Geometry check sheet. Reference: drawing and pictorial views, mm from the part's lowest x, y, z. Round coordinates to 2 decimals unless told otherwise and drop trailing zeros. Write each loop counter-clockwise with the first axis right and the second up, starting at its lowest first coordinate (ties: lowest second). Pieces come first, ordered by that corner, then holes.
Item 1: Section check B-B, the plane x = 14. Record the cut outline in (y, z) (1 decimal), plus the area to 3 significant figures.
Item 2: Section check C-C, the plane y = 65.5. State how many separate pieces and enclosed holes the cut face has.
Item 3: Material ranges on line 1 along Y through (x, z) = (19, 2.6) (1 decimal), recorded low to high.
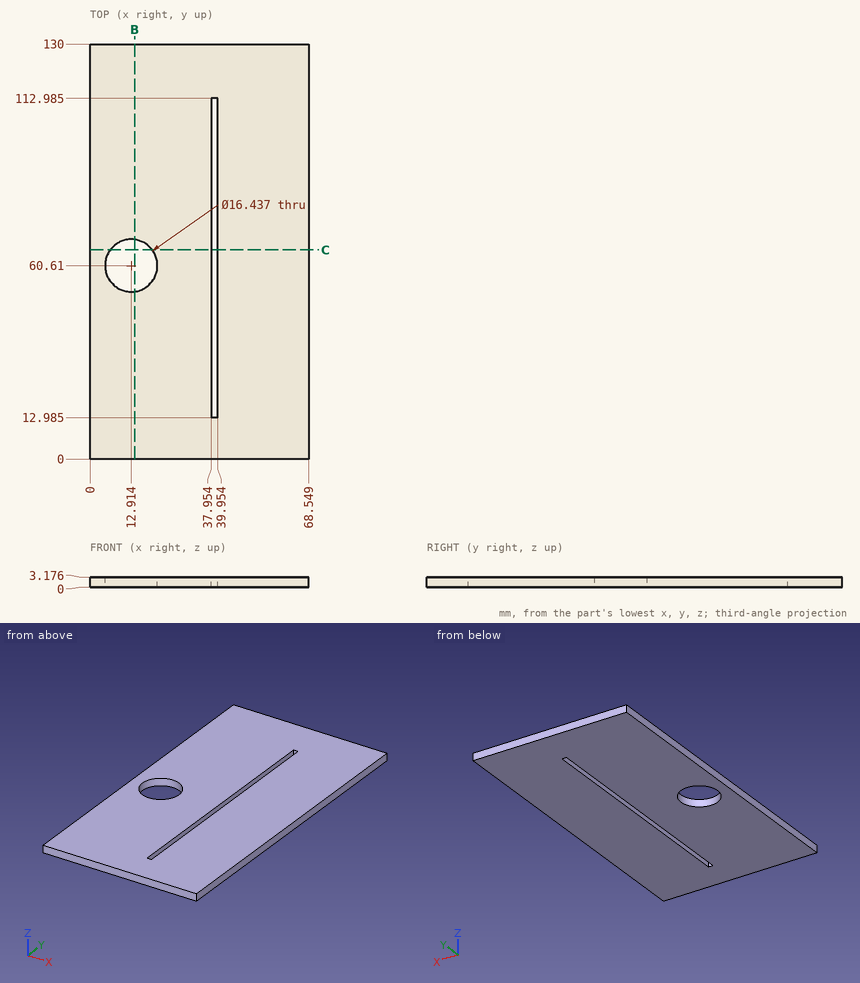
Values found:
1. outline: (0, 0) - (52.5, 0) - (52.5, 3.2) - (0, 3.2) - close; (68.8, 0) - (130, 0) - (130, 3.2) - (68.8, 3.2) - close
1. area: 361 mm2
2. separate pieces: 3
2. enclosed holes: 0
3. line 1: y = 0 to 55.1, 66.1 to 130
